Source: CAD feature listing. Evaluate the final solid. Frame: model axes, mm. Face numbers are marked on the shaded views. A direction names the side the tool comes from. Give positions to 0.01 mm unless a question says otherwise; leave off trailing zeros. Order: outer loops, then holes, each group sorted by start corner. A loop starts at its lowest first (then second) coordinate and runs counter-clockwise, first axis right, second up. Notation, with made-up numbers: (30, 52.5) - (53, 52.5) arc R18 cw to (53, 66.5) - close; hole circle Ø11 at (67.5, -29.5). An arc over 180 degrees is marked (long way). Write each question's results on one line, items separated by ' | '. Start each with the question number.
Item 1: Section D-D on x = 318. Output: boundary loops of the cut face in (y, z).
Item 2: Set-up query: the marked faces 1, 2, 3 and 4. Return all of +Z, -Z, +X, -X, +Y, -Y with unobstructed straight access to the full face (end or side cutting, diameter ignored); none if empty.
Item 3: Section B-B on x = 62. Output: boundary loops of the cut face in (y, z).
Item 4: Section C-C on y = 24. Output: boundary loops of the cut face in (x, z).
Item 5: Mould query, pull axis X, two halves, no side actions, for the marked faces 5, 6 and 7. Classes: released by +X, released by -X, zero draft, split by the parting line, or undercut.
Item 6: Contact query for flat-ended pins moving along their axis: pin 1 Ø8 at (x, z) = (137, -5) entering from +Y; pin 2 Ø10 at (x, y) = (108, 2.5) entering from +Z; pin 3 Ø3 at (y, z) = (32, -8.5) entering from -X; pin 4 Ø6 at (y, z) = (29.5, -17) entering from +X. Output: stop coordinate, or through.
Item 7: Line query: line 1 along X through (y, z) = (-19.25, 0); line 2 along X through (y, z) = (-13, 0); line 3 along X through (y, z) = (7, -10.5). Output: solid intervals per line, ascending.
Item 8: Section A-A on z = 0. State how many separate pieces and enclosed holes the cut face has, and give its area (3 significant figures).
```python
from build123d import *

# Parameters (mm, degrees)
SKETCH1_R           = 28
BOSS_EXTRUDE1_DEPTH = 247.1
SKETCH2_R           = 43.6
BOSS_EXTRUDE2_DEPTH = 24
SKETCH3_R           = 28
BOSS_EXTRUDE3_DEPTH = 89.8
SKETCH4_R           = 18.75
BOSS_EXTRUDE4_DEPTH = 28.9
CHAMFER1_SIZE       = 3
SKETCH5_W           = 193.8
SKETCH5_H           = 31.1
CUT_EXTRUDE1_DEPTH  = 54.45
CUT_EXTRUDE2_REACH  = 42.5
SKETCH6_R           = 6.25


with BuildPart() as part:
    # Sketch1 → Boss-Extrude1 (new body)
    with BuildSketch(Plane(origin=(0, 0, 0), x_dir=(0, 0, -1), z_dir=(1, 0, 0))):
        Circle(SKETCH1_R)
    extrude(amount=BOSS_EXTRUDE1_DEPTH)

    # Sketch2 → Boss-Extrude2 (add)
    with BuildSketch(Plane(origin=(247.1, 0, 0), x_dir=(0, 0, -1), z_dir=(1, 0, 0))):
        Circle(SKETCH2_R)
    extrude(amount=BOSS_EXTRUDE2_DEPTH)

    # Sketch3 → Boss-Extrude3 (add)
    with BuildSketch(Plane(origin=(271.1, 0, 0), x_dir=(0, 0, -1), z_dir=(1, 0, 0))):
        Circle(SKETCH3_R)
    extrude(amount=BOSS_EXTRUDE3_DEPTH)

    # Sketch4 → Boss-Extrude4 (add)
    with BuildSketch(Plane(origin=(360.9, 0, 0), x_dir=(0, 0, -1), z_dir=(1, 0, 0))):
        Circle(SKETCH4_R)
    extrude(amount=BOSS_EXTRUDE4_DEPTH)

    # Chamfer1
    chamfer1_edges = [part.edges().sort_by_distance(p)[0] for p in [
        (389.8, 0, 18.75),
    ]]
    chamfer(chamfer1_edges, length=CHAMFER1_SIZE)

    # Sketch5 → Cut-Extrude1 (cut, symmetric)
    with BuildSketch(Plane.XY):
        with Locations((112, 12.45)):
            Rectangle(SKETCH5_W, SKETCH5_H)
    extrude(amount=CUT_EXTRUDE1_DEPTH, both=True, mode=Mode.SUBTRACT)

    # Sketch6 → Cut-Extrude2 (cut, up to next)
    with BuildSketch(Plane(origin=(0, -3.1, 0), x_dir=(1, 0, 0), z_dir=(0, 1, 0)), mode=Mode.PRIVATE) as cut_extrude2_sk1:
        with Locations((62, 0)):
            Circle(SKETCH6_R)
    cut_extrude2_tool1 = extrude(cut_extrude2_sk1.sketch, amount=-CUT_EXTRUDE2_REACH, mode=Mode.PRIVATE) & part.part
    add(cut_extrude2_tool1.solids().sort_by_distance((62, -3.1, 0))[0], mode=Mode.SUBTRACT)
    # Sketch6 → Cut-Extrude2 (cut, up to next)
    with BuildSketch(Plane(origin=(0, -3.1, 0), x_dir=(1, 0, 0), z_dir=(0, 1, 0)), mode=Mode.PRIVATE) as cut_extrude2_sk2:
        with Locations((162, 0)):
            Circle(SKETCH6_R)
    cut_extrude2_tool2 = extrude(cut_extrude2_sk2.sketch, amount=-CUT_EXTRUDE2_REACH, mode=Mode.PRIVATE) & part.part
    add(cut_extrude2_tool2.solids().sort_by_distance((162, -3.1, 0))[0], mode=Mode.SUBTRACT)


solid = part.part
```
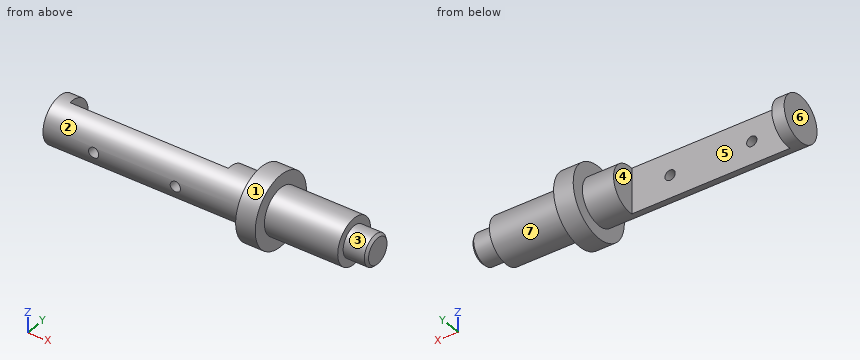
Evaluation:
1) outline: circle Ø56 at (0, 0)
2) face 1: +X, -X | face 2: -X | face 3: +X | face 4: +Z, -Z, +Y
3) outline: (-27.29, -6.25) arc R28 ccw to (-3.1, -27.83) - (-3.1, -6.25) - close; (-27.29, 6.25) - (-3.1, 6.25) - (-3.1, 27.83) arc R28 ccw to start
4) outline: (0, -14.42) - (15.1, -14.42) - (15.1, 14.42) - (0, 14.42) - close; (208.9, -14.42) - (247.1, -14.42) - (247.1, -36.4) - (271.1, -36.4) - (271.1, -14.42) - (360.9, -14.42) - (360.9, 14.42) - (271.1, 14.42) - (271.1, 36.4) - (247.1, 36.4) - (247.1, 14.42) - (208.9, 14.42) - close
5) face 5: undercut | face 6: released by -X | face 7: zero draft
6) pin 1: stops at y = -3.1 | pin 2: passes through | pin 3: stops at x = 247.1 | pin 4: stops at x = 271.1
7) line 1: x = 0 to 55.75, 68.25 to 155.75, 168.25 to 360.9 | line 2: x = 0 to 55.75, 68.25 to 155.75, 168.25 to 389.8 | line 3: x = 0 to 15.1, 208.9 to 389.8
8) separate pieces: 3 | enclosed holes: 0 | area: 15,400 mm^2
